Autodesk Inventor part; units mm, degrees
ref_plane "YZ Plane" through (0, 0, 0) normal (1, 0, 0) x (0, 1, 0)
ref_plane "XZ Plane" through (0, 0, 0) normal (0, 1, 0) x (-1, 0, 0)
ref_plane "XY Plane" through (0, 0, 0) normal (0, 0, 1) x (1, 0, 0)
sketch "Sketch1" plane through (0, 0, 0) normal (0, 0, 1) x (1, 0, 0)
  circle A0 centre (46.0449, -16.759) radius 4 construction
  spline S0 degree 3 poles (32.2129, 20.8318) (30.525, 21.8832) (29.0415, 23.2334) (25.9174, 26.8655) (24.5253, 29.2164) (23.4072, 31.3618) knots 0 0 0 0 0.391133 0.391133 0.939024 0.939024 0.939024 0.939024 construction
  arc A1 (50.7434, -18.4691) -> (41.3465, -15.0489) centre (46.0449, -16.759) ccw
  circle A2 centre (46.0449, -16.759) radius 1.5
  arc A3 (5.4493, -30.9044) -> (24.0394, -20.1714) centre (0, 0) ccw
  arc A4 (26.086, -47.2813) -> (50.7434, -18.4691) centre (0, 0) ccw
  arc A5 (40.5335, -17.1182) -> (41.3465, -15.0489) centre (0, 0) ccw
  circle A6 centre (0, 0) radius 49 construction
  line L0 (46.0449, -16.759) -> (0, 0) construction
  line L1 (0, 0) -> (49, 0) construction
  line L2 (5.4493, -30.9044) -> (0, 0) construction
  line L3 (24.0394, -20.1714) -> (0, 0) construction
  line L4 (24.0394, -20.1714) -> (24.8935, -20.8881)
  line L5 (0, 0) -> (15.6906, -27.1769) construction
  arc A7 (24.8935, -20.8881) -> (40.5335, -17.1182) centre (31.3214, -13.2277) ccw
  arc A8 (5.4493, -30.9044) -> (13.7408, -45.1235) centre (46.0449, -16.759) ccw
  arc A9 (13.7408, -45.1235) -> (26.086, -47.2813) centre (21.2552, -38.5255) ccw
  point P0 (33.706, -28.2827)
  dimension "d2" = 62.7624
  dimension "d3" = 10
  dimension "d4" = 3
  dimension "d5" = 8
  dimension "d42" = 98
  dimension "d45" = 20
  dimension "d46" = 40
  dimension "d47" = 20
  dimension "d48" = 60
  dimension "d49" = 10
  dimension "d51" = 10
extrude "Extrusion1" add sketch "Sketch1" along normal blind 4
sketch "Sketch10" plane through (0, 0, 4) normal (0, 0, 1) x (1, 0, 0)
  arc A0 (26.086, -47.2813) -> (50.7434, -18.4691) centre (0, 0) ccw
  arc A1 (47.7831, -25.1551) -> (33.0704, -42.689) centre (57.4533, -48.2091) ccw
  arc A2 (40.5335, -17.1182) -> (41.3465, -15.0489) centre (0, 0) ccw
  line L0 (57.4533, -48.2091) -> (0, 0) construction
  line L1 (0, 0) -> (52.518, 0) construction
  dimension "d54" = 40
  dimension "d55" = 25
  dimension "d56" = 75
extrude "Extrusion9" cut sketch "Sketch10" against normal blind 10
fillet "Fillet8" radius 10 2 edges at (47.7831, -25.1551, 2) (33.0704, -42.689, 2)
equation "\"d51\" = d49"
properties part number "launcher.latch"
Model file for the job. Use its own axes, mm. Coordinates: 2 decimals unless noted, no trailing zeros. Order: outer loops, then holes, each group sorted by start corner. A loop starts at its lowest first (then second) coordinate and runs counter-clockwise, first axis right, second up. Notation, with made-up numbers: M 42.5,74 L 61.5,74 A17 ccw 61.5,89 Z; hole C -6,-11.75 d3. An arc over 180 degrees is marked long. Return JSON: item names as keys, results as strings.
1. Saw through at B-B (y = -27.5). Give the cut face in (x, z), and give its area (3 significant figures).
Ans:
{"outline": "M 15.12,0 L 43.45,0 L 43.45,4 L 15.12,4 Z", "area": "113 mm^2"}
2. Flat gauge pins, fed straight in: pin 1 (2.5 mm diameter, centred on x = 46.04, y = -16.76, fed in from -Z); pin 2 (1.5 mm diameter, centred on x = 32, z = 2, fed in from +Y); pin 3 (2 mm diameter, centred on y = -38, z = 2, fed in from -X). Where does each tip first touch, or does it go through?
Ans:
{"pin 1": "through", "pin 2": "y = -23.13", "pin 3": "x = 8.12"}
3. Saw through at A-A (x = 18.5). Give the cut face in (y, z), and give its area (3 significant figures).
Ans:
{"outline": "M -48.14,0 L -25.35,0 L -25.35,4 L -48.14,4 Z", "area": "91.2 mm^2"}
4. Drill centre lines: probe 1 along Y at (x, z) = (45.5, 2.6); probe 2 along X at (y, z) = (-43, 3.05); probe 3 along X at (y, z) = (-25, 2.65). Where is each one in solid material? Low to high.
Ans:
{"probe 1": "-26.24 to -18.16, -15.36 to -11.79", "probe 2": "11.99 to 32.11", "probe 3": "18.97 to 47.13"}
5. Pull direction Y, two halves, no side cores. Call faces 1 (the face through (28, -30, 4)), 2 (the face through (33.79, -22.92, 1.97)), 3 (the face through (47.43, -16.18, 1.97)): +Y half, -Y half, draft (parallel to the pull), parting line (faces both ways), or undercut.
Ans:
{"face 1": "draft", "face 2": "+Y half", "face 3": "undercut"}
